Geometry: final body of the model. Coordinates: model frame, mm. Give positions to 0.01 mm unless a question says otherwise; leave off trailing zeros. Answer in a Markdown table with one row per item.
Autodesk Inventor part; units mm, degrees
ref_plane "YZ Plane" through (0, 0, 0) normal (1, 0, 0) x (0, 1, 0)
ref_plane "XZ Plane" through (0, 0, 0) normal (0, 1, 0) x (-1, 0, 0)
ref_plane "XY Plane" through (0, 0, 0) normal (0, 0, 1) x (1, 0, 0)
sketch "Sketch1" plane through (0, 0, 0) normal (0, 0, 1) x (1, 0, 0)
  line L0 (0, 0) -> (148.627, 0)
  line L1 (148.627, 0) -> (148.627, 10)
  line L2 (148.627, 10) -> (0, 10)
  line L3 (0, 10) -> (0, 0)
  dimension "d0" = 148.627
  dimension "d1" = 10
extrude "Extrusion1" add sketch "Sketch1" along normal blind 12
sketch "Sketch2" plane through (0, 0, 12) normal (0, 0, 1) x (1, 0, 0)
  arc A0 (4.1138, 10) -> (2.9206, 14.6043) centre (-12.3652, 8.1863) ccw
  arc A1 (2.9206, 14.6043) -> (1.1932, 14.6043) centre (2.0569, -7.3787) ccw
  arc A2 (1.1932, 14.6043) -> (0, 10) centre (16.479, 8.1863) ccw
  line L0 (0, 0) -> (148.627, 0)
  line L1 (148.627, 0) -> (148.627, 10)
  line L2 (148.627, 10) -> (0, 10)
  line L3 (0, 10) -> (0, 0)
  line L4 (148.627, 10) -> (0, 10)
  line L5 (0, 10) -> (4.1138, 10)
  dimension "d4" = 16.5785
  dimension "d5" = 16.5785
  dimension "d6" = 22
  dimension "d7" = 28.8442
  dimension "d8" = 1.1932
  dimension "d9" = 6.418
  dimension "d10" = 4.6043
  dimension "d11" = 1.1932
extrude "Extrusion2" add sketch "Sketch2" against normal blind 12 contours L2 A2 A1 A0
pattern_linear "Rectangular Pattern1" count 24 spacing 6.2832 along (1, 0, 0) of "Extrusion2"
properties part number "Cremallera"
Q1. First-contact query: pin 1 (1.1 mm diameter, centred on x = 30, z = 9, fed in from +Y); pin 2 (3 mm diameter, centred on y = 2.5, z = 7.5, fed in from -X). Flat tips, straight axial feed; report the tip coordinate or a pass-through.
Check values:
| item | result |
|---|---|
| pin 1 | y = 10 |
| pin 2 | x = 0 |
Q2. Material intervals for line 1 along Y through (x, z) = (80.5, 9.25); line 2 along Y through (x, z) = (71, 3.25), sorted ascending.
Check values:
| item | result |
|---|---|
| line 1 | 0 to 10 |
| line 2 | 0 to 14.62 |
Q3. Draft query along X for faces 1 (the flat face through (73, 6, 12)), 2 (the flat face through (148.627, 5, 6)), 3 (the cylindrical face through (75.84, 12.38, 6.08)). Return one class per face: pulls with the +X half, pulls with the -X half, needs draft (parallel to the pull), parting line crosses it, or undercut.
Check values:
| item | result |
|---|---|
| face 1 | needs draft |
| face 2 | pulls with the +X half |
| face 3 | undercut |
Q4. Cut plane A-A (y = 12). Give the number of separate pieces and of enclosed holes in the cut face, and give its area (3 significant figures).
Check values:
| item | result |
|---|---|
| separate pieces | 24 |
| enclosed holes | 0 |
| area | 986 mm² |
